Check sheet for the modelled part. Datum: model origin and axes. Units: mm. A direction names the side the tool comes from. Give positions to 0.01 mm unless a question says otherwise; leave off trailing zeros. Write each question's results on one line, items separated by ' | '. Start each with the question number.
Item 1: Scan lines: line 1 along Z through (x, y) = (3.5, 44); line 2 along Z through (x, y) = (9, 52); line 3 along Z through (x, y) = (15, 38). Record each from-to range of solid material in increasing order.
Item 2: Access from +Z, -Z, +X, -X, +Y, -Y to the whole of each face (thin tool, end or side, straight path). Record for faces 4 (the face through (6.35, 53, 41)), 5 (the face through (22, 62.5, 117)), 6 (the face through (6, 37.1, 134)), 7 (the face through (37.69, 17.21, 231.12)).
Item 3: Mould release check, pull along Z, two halves, no side actions. Record for faces 1 (the face through (36, 46, 224.68)), 2 (the face through (9.15, 16.34, 231.12)), 3 (the face through (29.557, 6.261, 22.36)): pulls with the +Z half, pulls with the -Z half, needs draft (parallel to the pull), parting line crosses it, or undercut.
Item 4: Gauge pin test, flat ends, axial feed: pin 1 Ø1.3 at (y, z) = (52.5, 196.5) entering from -X; pin 2 Ø3 at (x, y) = (8.5, 47) entering from +Z; pin 3 Ø4 at (x, z) = (19.12, 180.14) entering from +Y. Record the tip position at first contact, or that the pin passes through.
from build123d import *

# Parameters (mm, degrees)
SKETCH1_W           = 44.45
SKETCH1_H           = 62.5
BOSS_EXTRUDE1_DEPTH = 237.38
CUT_EXTRUDE1_DEPTH  = 238.38
CUT_EXTRUDE2_DEPTH  = 32
CUT_EXTRUDE3_DEPTH  = 12.7
SKETCH4_R           = 3.175
CUT_EXTRUDE4_DEPTH  = 6.35
CUT_EXTRUDE5_DEPTH  = 25.4
SKETCH6_R           = 7.9375
CUT_EXTRUDE6_DEPTH  = 12.7


with BuildPart() as part:
    # Sketch1 → Boss-Extrude1 (new body)
    with BuildSketch(Plane.XY):
        with Locations((22.225, 31.25)):
            Rectangle(SKETCH1_W, SKETCH1_H)
    extrude(amount=BOSS_EXTRUDE1_DEPTH)

    # Sketch2 → Cut-Extrude1 (cut, through all)
    with BuildSketch(Plane.XY.offset(237.38)):
        with BuildLine():
            ThreePointArc((14.225, 32.5), (22.225, 24.5), (30.225, 32.5))
            ThreePointArc((30.225, 32.5), (22.225, 40.5), (14.225, 32.5))
        make_face()
    extrude(amount=-CUT_EXTRUDE1_DEPTH, mode=Mode.SUBTRACT)

    # Sketch2_4 → Cut-Extrude2 (cut)
    with BuildSketch(Plane.XY.offset(237.38)):
        with BuildLine():
            ThreePointArc((8.225, 32.5), (22.225, 18.5), (36.225, 32.5))
            ThreePointArc((36.225, 32.5), (22.225, 46.5), (8.225, 32.5))
        make_face()
        with BuildLine():
            ThreePointArc((30.225, 32.5), (22.225, 40.5), (14.225, 32.5))
            ThreePointArc((14.225, 32.5), (22.225, 24.5), (30.225, 32.5))
        make_face(mode=Mode.SUBTRACT)
    extrude(amount=-CUT_EXTRUDE2_DEPTH, mode=Mode.SUBTRACT)

    # Sketch2_5 → Cut-Extrude3 (cut)
    with BuildSketch(Plane.XY.offset(237.38)):
        with BuildLine():
            ThreePointArc((11.539971157, 45.935028843), (8.789971157, 48.685028843), (6.039971157, 45.935028843))
            ThreePointArc((6.039971157, 45.935028843), (8.789971157, 43.185028843), (11.539971157, 45.935028843))
        make_face()
        with BuildLine():
            ThreePointArc((24.975, 51.5), (22.225, 54.25), (19.475, 51.5))
            ThreePointArc((19.475, 51.5), (22.225, 48.75), (24.975, 51.5))
        make_face()
        with BuildLine():
            ThreePointArc((38.410028843, 45.935028843), (35.660028843, 48.685028843), (32.910028843, 45.935028843))
            ThreePointArc((32.910028843, 45.935028843), (35.660028843, 43.185028843), (38.410028843, 45.935028843))
        make_face()
        with BuildLine():
            ThreePointArc((38.410028843, 19.064971157), (35.660028843, 21.814971157), (32.910028843, 19.064971157))
            ThreePointArc((32.910028843, 19.064971157), (35.660028843, 16.314971157), (38.410028843, 19.064971157))
        make_face()
        with BuildLine():
            ThreePointArc((24.975, 13.5), (22.225, 16.25), (19.475, 13.5))
            ThreePointArc((19.475, 13.5), (22.225, 10.75), (24.975, 13.5))
        make_face()
        with BuildLine():
            ThreePointArc((11.539971157, 19.064971157), (8.789971157, 21.814971157), (6.039971157, 19.064971157))
            ThreePointArc((6.039971157, 19.064971157), (8.789971157, 16.314971157), (11.539971157, 19.064971157))
        make_face()
    extrude(amount=-CUT_EXTRUDE3_DEPTH, mode=Mode.SUBTRACT)

    # Sketch4 → Cut-Extrude4 (cut)
    with BuildSketch(Plane.ZY):
        with Locations((157.144917681, 35.325)):
            Circle(SKETCH4_R)
        with Locations((157.144917681, 54.375)):
            Circle(SKETCH4_R)
        with BuildLine():
            ThreePointArc((41.4, 55.1), (39.763489429, 54.315991319), (39.348920282, 52.549364905))
            ThreePointArc((39.348920282, 52.549364905), (40.084008681, 51.363489429), (41.4, 50.9))
            ThreePointArc((41.4, 50.9), (43.5, 53), (41.4, 55.1))
        make_face()
        with BuildLine():
            ThreePointArc((13.3, 53), (13.91507576, 51.51507576), (15.4, 50.9))
            ThreePointArc((15.4, 50.9), (17.5, 53), (15.4, 55.1))
            ThreePointArc((15.4, 55.1), (13.91507576, 54.48492424), (13.3, 53))
        make_face()
        with BuildLine():
            ThreePointArc((221.98, 50.9), (224.08, 53), (221.98, 55.1))
            ThreePointArc((221.98, 55.1), (220.343489429, 54.315991319), (219.928920282, 52.549364905))
            ThreePointArc((219.928920282, 52.549364905), (220.664008681, 51.363489429), (221.98, 50.9))
        make_face()
        with BuildLine():
            ThreePointArc((193.88, 53), (194.49507576, 51.51507576), (195.98, 50.9))
            ThreePointArc((195.98, 50.9), (198.08, 53), (195.98, 55.1))
            ThreePointArc((195.98, 55.1), (194.49507576, 54.48492424), (193.88, 53))
        make_face()
        with BuildLine():
            ThreePointArc((219.928920282, 12.450635095), (220.343489429, 10.684008681), (221.98, 9.9))
            ThreePointArc((221.98, 9.9), (224.08, 12), (221.98, 14.1))
            ThreePointArc((221.98, 14.1), (220.664008681, 13.636510571), (219.928920282, 12.450635095))
        make_face()
        with BuildLine():
            ThreePointArc((193.88, 12), (194.49507576, 10.51507576), (195.98, 9.9))
            ThreePointArc((195.98, 9.9), (198.08, 12), (195.98, 14.1))
            ThreePointArc((195.98, 14.1), (194.49507576, 13.48492424), (193.88, 12))
        make_face()
        with BuildLine():
            ThreePointArc((13.3, 12), (13.91507576, 10.51507576), (15.4, 9.9))
            ThreePointArc((15.4, 9.9), (17.5, 12), (15.4, 14.1))
            ThreePointArc((15.4, 14.1), (13.91507576, 13.48492424), (13.3, 12))
        make_face()
        with BuildLine():
            ThreePointArc((39.348920282, 12.450635095), (39.763489429, 10.684008681), (41.4, 9.9))
            ThreePointArc((41.4, 9.9), (43.5, 12), (41.4, 14.1))
            ThreePointArc((41.4, 14.1), (40.084008681, 13.636510571), (39.348920282, 12.450635095))
        make_face()
    extrude(amount=-CUT_EXTRUDE4_DEPTH, mode=Mode.SUBTRACT)

    # Sketch5 → Cut-Extrude5 (cut)
    with BuildSketch(Plane(origin=(0, 62.5, 0), x_dir=(1, 0, 0), z_dir=(0, 1, 0))):
        with BuildLine():
            ThreePointArc((9.425, -134.144917681), (6.125, -130.844917681), (2.825, -134.144917681))
            ThreePointArc((2.825, -134.144917681), (6.125, -137.444917681), (9.425, -134.144917681))
        make_face()
        with BuildLine():
            ThreePointArc((22.425, -134.144917681), (19.125, -130.844917681), (15.825, -134.144917681))
            ThreePointArc((15.825, -134.144917681), (19.125, -137.444917681), (22.425, -134.144917681))
        make_face()
        with BuildLine():
            ThreePointArc((9.425, -180.144917681), (6.125, -176.844917681), (2.825, -180.144917681))
            ThreePointArc((2.825, -180.144917681), (6.125, -183.444917681), (9.425, -180.144917681))
        make_face()
        with BuildLine():
            ThreePointArc((22.425, -180.144917681), (19.125, -176.844917681), (15.825, -180.144917681))
            ThreePointArc((15.825, -180.144917681), (19.125, -183.444917681), (22.425, -180.144917681))
        make_face()
    extrude(amount=-CUT_EXTRUDE5_DEPTH, mode=Mode.SUBTRACT)

    # Sketch6 → Cut-Extrude6 (cut)
    with BuildSketch(Plane.XZ):
        with Locations((22.225, 211.98)):
            Circle(SKETCH6_R)
        with Locations((22.225, 25.4)):
            Circle(SKETCH6_R)
    extrude(amount=-CUT_EXTRUDE6_DEPTH, mode=Mode.SUBTRACT)


solid = part.part
Answer sheet:
1) line 1: z = 0 to 132.15, 136.14 to 178.15, 182.14 to 237.38 | line 2: z = 0 to 132.52, 135.76 to 178.52, 181.76 to 237.38 | line 3: z = 0 to 205.38
2) face 4: -X | face 5: +Z, -Z, +X, -X, +Y | face 6: +Y | face 7: +Z
3) face 1: pulls with the +Z half | face 2: needs draft | face 3: undercut
4) pin 1: stops at x = 6.35 | pin 2: stops at z = 224.68 | pin 3: stops at y = 26.34
